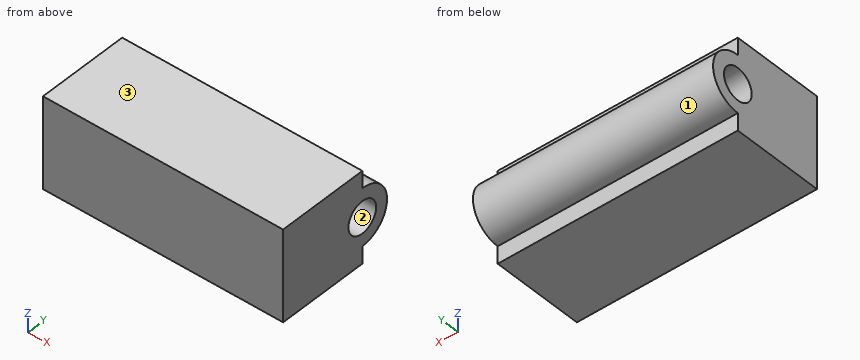
```python
from build123d import *

# Parameters (mm, degrees)
SKETCH_1_W      = 210
SKETCH_1_H      = 80
EXTRUDE_1_DEPTH = 50
SKETCH_2_R      = 14
EXTRUDE_2_DEPTH = 210


with BuildPart() as part:
    # 草图1 → 凸台-拉伸1 (new body)
    with BuildSketch(Plane(origin=(0, 0, 0), x_dir=(1, 0, 0), z_dir=(0, 1, 0))):
        Rectangle(SKETCH_1_W, SKETCH_1_H)
    extrude(amount=EXTRUDE_1_DEPTH)

    # 草图2 → 凸台-拉伸2 (add)
    with BuildSketch(Plane.ZY.offset(105)):
        with BuildLine():
            Line((25, 80), (40, 80))
            Line((40, 80), (40, 50))
            Line((40, 50), (-40, 50))
            Line((-40, 50), (-40, 80))
            Line((-40, 80), (-25, 80))
            ThreePointArc((-25, 80), (0, 105), (25, 80))
        make_face()
        with Locations((0, 80)):
            Circle(SKETCH_2_R, mode=Mode.SUBTRACT)
    extrude(amount=-EXTRUDE_2_DEPTH)


solid = part.part
```
Work out the finished part from the listing and answer in its coordinate system (mm). Face numbers are marked on the shaded views. Round coordinates to 2 decimals unless told otherwise and drop trailing zeros. Loops run counter-clockwise (first coordinate to the right, second up) from the corner with the lowest first, then second, coordinate; pieces in that order, holes last.
(1) The part is cut by section C-C, the plane y = 85. Give the vertices of the cut face in (x, z).
Computed values:
outline: (-105, -24.49) - (105, -24.49) - (105, -13.08) - (-105, -13.08) - close; (-105, 13.08) - (105, 13.08) - (105, 24.49) - (-105, 24.49) - close
(2) Find the intervals of material crossed by L1, parallel to Y at x = 49, z = 0; L2, parallel to Y at x = 5, z = 9.5; L3, parallel to Z at x = 1, y = 83, in increasing order.
Computed values:
L1: y = 0 to 66, 94 to 105
L2: y = 0 to 69.72, 90.28 to 103.12
L3: z = -24.82 to -13.67, 13.67 to 24.82
(3) The part is cut by section B-B, the plane x = 59. Give the vertices of the cut face in (y, z).
Computed values:
outline: (0, -40) - (80, -40) - (80, -25) arc R25 ccw to (80, 25) - (80, 40) - (0, 40) - close; hole circle Ø28 at (80, 0)
(4) The part is cut by section D-D, the plane z = 23. Give the vertices of the cut face in (x, y).
Computed values:
outline: (-105, 0) - (105, 0) - (105, 89.8) - (-105, 89.8) - close
(5) Each of these flat-tipped pins is pushed along its axis until it touches: P1, Ø12, axis at x = -50, z = 32, coming from the +Y side; P2, Ø25, axis at y = 80, z = 0, coming from the -X side; P3, Ø10, axis at x = 59, z = -28.5, coming from the -Y side; P4, Ø3, axis at x = 26, z = -23.5, coming from the +Y side. Where does it stop, or does it pass through?
Computed values:
P1: stops at y = 80
P2: passes through
P3: stops at y = 0
P4: stops at y = 91.87
(6) The mould has two halves that part along Z. Classify the marked faces 1, 2 and 3: pulls with the +Z half, pulls with the -Z half, needs draft (parallel to the pull), parting line crosses it, or undercut.
Computed values:
face 1: parting line crosses it
face 2: undercut
face 3: pulls with the +Z half
(7) The part is cut by section A-A, the plane z = 0. Give the vertices of the cut face in (x, y).
Computed values:
outline: (-105, 0) - (105, 0) - (105, 66) - (-105, 66) - close; (-105, 94) - (105, 94) - (105, 105) - (-105, 105) - close
